```python
from build123d import *

# Parameters (mm, degrees)
BOSS_EXTRU_1_DEPTH      = 1000
ESQUISSE2_R             = 3.05
ENL_V_MAT_EXTRU_1_DEPTH = 500
ESQUISSE3_R             = 2.05
ENL_V_MAT_EXTRU_2_DEPTH = 5
ESQUISSE4_R             = 3.1
ENL_V_MAT_EXTRU_3_DEPTH = 310


with BuildPart() as part:
    # Esquisse1 → Boss.-Extru.1 (new body)
    with BuildSketch(Plane.XY):
        with BuildLine():
            Line((0, 150), (0, 148))
            ThreePointArc((0, 148), (-104.651803616, 104.651803616), (-148, 0))
            Line((-148, 0), (-148, -20))
            Line((-148, -20), (-150, -20))
            Line((-150, -20), (-150, 0))
            ThreePointArc((-150, 0), (-106.066017178, 106.066017178), (0, 150))
        make_face()
    extrude(amount=BOSS_EXTRU_1_DEPTH)

    # Esquisse2 → Enlèv. mat.-Extru.1 (cut)
    with BuildSketch(Plane.ZY.offset(150)):
        with Locations(Location((10, -10, 0), (0, 0, 270))):
            Circle(ESQUISSE2_R)
        with Locations(Location((990, -10, 0), (0, 0, 270))):
            Circle(ESQUISSE2_R)
    extrude(amount=-ENL_V_MAT_EXTRU_1_DEPTH, mode=Mode.SUBTRACT)

    # Esquisse3 → Enlèv. mat.-Extru.2 (cut)
    with BuildSketch(Plane.ZY.offset(150)):
        with Locations(Location((4, -4, 0), (0, 0, 270))):
            Circle(ESQUISSE3_R)
        with Locations(Location((16, -4, 0), (0, 0, 270))):
            Circle(ESQUISSE3_R)
        with Locations(Location((4, -16, 0), (0, 0, 270))):
            Circle(ESQUISSE3_R)
        with Locations(Location((16, -16, 0), (0, 0, 270))):
            Circle(ESQUISSE3_R)
        with Locations(Location((494, -4, 0), (0, 0, 270))):
            Circle(ESQUISSE3_R)
        with Locations(Location((506, -4, 0), (0, 0, 270))):
            Circle(ESQUISSE3_R)
        with Locations(Location((494, -16, 0), (0, 0, 270))):
            Circle(ESQUISSE3_R)
        with Locations(Location((506, -16, 0), (0, 0, 270))):
            Circle(ESQUISSE3_R)
        with Locations(Location((984, -4, 0), (0, 0, 270))):
            Circle(ESQUISSE3_R)
        with Locations(Location((996, -4, 0), (0, 0, 270))):
            Circle(ESQUISSE3_R)
        with Locations(Location((984, -16, 0), (0, 0, 270))):
            Circle(ESQUISSE3_R)
        with Locations(Location((996, -16, 0), (0, 0, 270))):
            Circle(ESQUISSE3_R)
    extrude(amount=-ENL_V_MAT_EXTRU_2_DEPTH, mode=Mode.SUBTRACT)

    # Symétrie2: part across plane


with BuildPart() as part_1:
    add(part.part)
    add(part.part.mirror(Plane(origin=(0, 150, 1000), x_dir=(0, 0, 1), z_dir=(-1, 0, 0))))

    # Esquisse4 → Enlèv. mat.-Extru.3 (cut)
    with BuildSketch(Plane.ZY.offset(150)):
        with Locations((500, -20)):
            Circle(ESQUISSE4_R)
    extrude(amount=-ENL_V_MAT_EXTRU_3_DEPTH, mode=Mode.SUBTRACT)


solid = part_1.part
```
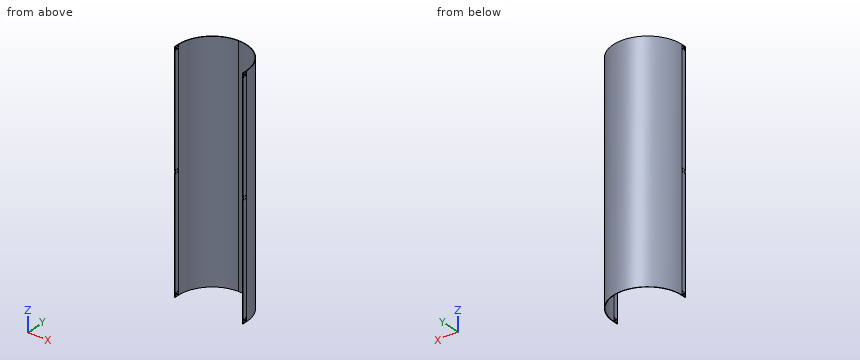
For this review, take the finished solid that the model builds, in its own axes (mm). Round coordinates to 2 decimals unless told otherwise and drop trailing zeros. Write each loop counter-clockwise with the first axis right and the second up, starting at its lowest first coordinate (ties: lowest second). Pieces come first, ordered by that corner, then holes. Notation, with made-up numbers: (5.25, -2) - (11.25, -2) arc R18 cw to (11.25, 11) - close; hole circle Ø6 at (-32, -26). An arc over 180 degrees is marked (long way). Put each result on its own line as item: value.
Q1. We need section A-A (y = 26). Give the boundary of the cut face in (x, z).
Solved:
outline: (-147.73, 0) - (-145.7, 0) - (-145.7, 1000) - (-147.73, 1000) - close; (145.7, 0) - (147.73, 0) - (147.73, 1000) - (145.7, 1000) - close
Q2. Insertion check: pin 1 Ø3.5 at (y, z) = (-4, 4) entering from -X; pin 2 Ø12 at (y, z) = (17, 419) entering from +X; pin 3 Ø6 at (y, z) = (97.5, 738) entering from -X; pin 4 Ø1 at (x, z) = (6, 279.5) entering from +Y. Each pin has a flat end and moves straight along its axis. Give the tip position at first contact, or say it passes through.
Solved:
pin 1: passes through
pin 2: stops at x = 149.6
pin 3: stops at x = -116.49
pin 4: stops at y = 149.9
Q3. We need section B-B (z = 156.5). Give the boundary of the cut face in (x, y).
Solved:
outline: (-150, -20) - (-148, -20) - (-148, 0) arc R148 cw to (148, 0) - (148, -20) - (150, -20) - (150, 0) arc R150 ccw to (-150, 0) - close
Q4. We need section D-D (x = -29.5). Give the boundary of the cut face in (y, z).
Solved:
outline: (145.03, 0) - (147.07, 0) - (147.07, 1000) - (145.03, 1000) - close
Q5. Wall thickness on probe 1 along X at (y, z) = (-7, 604.5); probe 2 along X at (y, z) = (88, 570); probe 3 along Y at (x, z) = (-17.5, 817): over which ranges is each line inside the solid? List them lowest first.
Solved:
probe 1: x = -150 to -148, 148 to 150
probe 2: x = -121.47 to -119, 119 to 121.47
probe 3: y = 146.96 to 148.98
